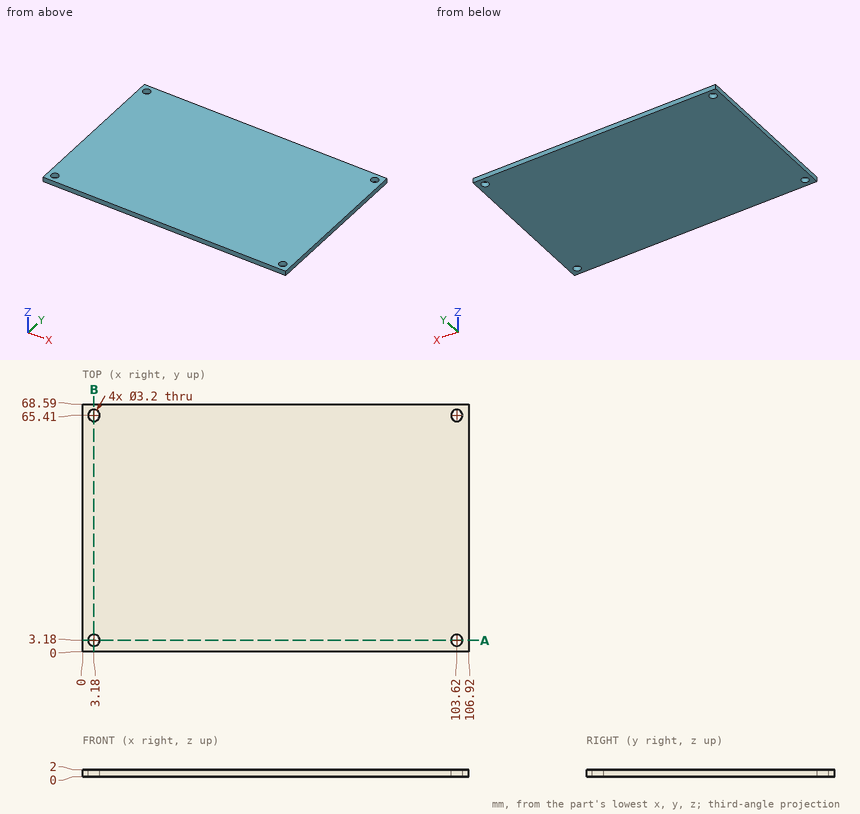
Geometry check sheet. Reference: drawing and pictorial views, mm from the part's lowest x, y, z. Give positions to 0.01 mm unless a question says otherwise; leave off trailing zeros. Loops run counter-clockwise (first coordinate to the right, second up) from the corner with the lowest first, then second, coordinate; pieces in that order, holes last. Notation, with made-up numbers: M 4.5,26.5 L 46.5,26.5 A33 ccw 46.5,62.5 Z; hole C -4.75,3 d8. An arc over 180 degrees is marked long. Use a Markdown table: item, result. Add a question column.
Q1. Scan lines: line 1 along Y through (x, z) = (103.62, 1.5); line 2 along X through (y, z) = (65.41, 1.4). Record each from-to range of solid material in increasing order. Write a range as [from, to].
Q2. Sectioned sample at B-B, the plane x = 3.18. Record the cut outline in (y, z), then the cut area to 3 significant figures.
Q3. Go/stop test with a flat-tipped pin: pin 1 (3 mm diameter, centred on x = 103.62, y = 65.41, fed in from -Z). Record where the tip stops, or that it passes through.
Q4. Sectioned sample at A-A, the plane y = 3.18. Record the cut outline in (x, z).
Verdict:
| question | item | result |
|---|---|---|
| 1 | line 1 | [0, 1.58], [4.78, 63.81], [67.01, 68.59] |
| 1 | line 2 | [0, 1.58], [4.78, 102.02], [105.22, 106.92] |
| 2 | outline | M 0,0 L 1.58,0 L 1.58,2 L 0,2 Z; M 4.78,0 L 63.81,0 L 63.81,2 L 4.78,2 Z; M 67.01,0 L 68.59,0 L 68.59,2 L 67.01,2 Z |
| 2 | area | 124 mm^2 |
| 3 | pin 1 | through |
| 4 | outline | M 0,0 L 1.58,0 L 1.58,2 L 0,2 Z; M 4.78,0 L 102.02,0 L 102.02,2 L 4.78,2 Z; M 105.22,0 L 106.92,0 L 106.92,2 L 105.22,2 Z |
